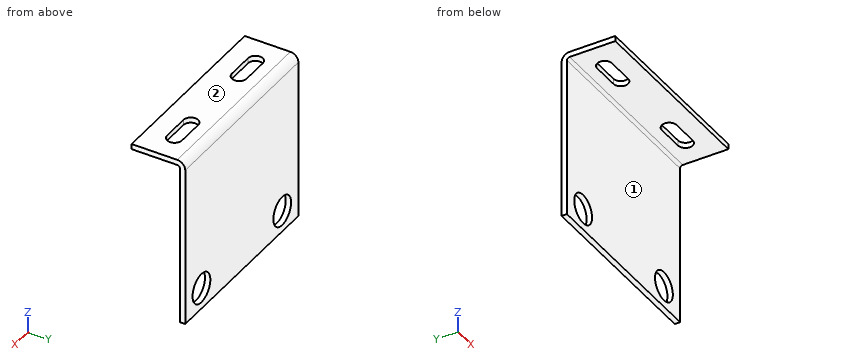
from build123d import *

# Parameters (mm, degrees)
SKETCH_1_W             = 70
SKETCH_1_H             = 60
SM_BASE_FLANGE_1_DEPTH = 2
SM_EDGE_FLANGE_1_DEPTH = 70
CUT_EXTRUDE_1_DEPTH    = 10
SKETCH_13_R            = 5.5
CUT_EXTRUDE_2_DEPTH    = 10


# Sheet-metal steps are written as plain solids
with BuildPart() as part:
    # Sketch 1 → 基体-法兰1 (new body)
    with BuildSketch(Plane(origin=(0, 0, 0), x_dir=(1, 0, 0), z_dir=(0, 1, 0))):
        with Locations((35, 30)):
            Rectangle(SKETCH_1_W, SKETCH_1_H)
    extrude(amount=-SM_BASE_FLANGE_1_DEPTH)

    # 边线-法兰1 section (across the edge) → 边线-法兰1 (add)
    with BuildSketch(Plane(origin=(70, -2, 1), x_dir=(0, 0, -1), z_dir=(-1, 0, 0))):
        with BuildLine():
            Line((-2, 1), (-2, 18))
            Line((-2, 18), (0, 18))
            Line((0, 18), (0, 1))
            ThreePointArc((0, 1), (0.292893219, 0.292893219), (1, 0))
            Line((1, 0), (1, -2))
            ThreePointArc((1, -2), (-1.121320344, -1.121320344), (-2, 1))
        make_face()
    extrude(amount=SM_EDGE_FLANGE_1_DEPTH)

    # 草图12 → 切除-拉伸1 (cut)
    with BuildSketch(Plane(origin=(0, 0, 1), x_dir=(-1, 0, 0), z_dir=(0, 0, -1))):
        with BuildLine():
            Line((-60, -7.25), (-50, -7.25))
            ThreePointArc((-50, -7.25), (-47.25, -10), (-50, -12.75))
            Line((-50, -12.75), (-60, -12.75))
            ThreePointArc((-60, -12.75), (-62.75, -10), (-60, -7.25))
        make_face()
        with BuildLine():
            Line((-10, -7.25), (-20, -7.25))
            ThreePointArc((-20, -7.25), (-22.75, -10), (-20, -12.75))
            Line((-20, -12.75), (-10, -12.75))
            ThreePointArc((-10, -12.75), (-7.25, -10), (-10, -7.25))
        make_face()
    extrude(amount=-CUT_EXTRUDE_1_DEPTH, mode=Mode.SUBTRACT)

    # 草图13 → 切除-拉伸2 (cut)
    with BuildSketch(Plane(origin=(0, 0, 0), x_dir=(1, 0, 0), z_dir=(0, 1, 0))):
        with Locations(Location((10, 52, 0), (0, 0, 270))):
            Circle(SKETCH_13_R)
        with Locations(Location((60, 52, 0), (0, 0, 270))):
            Circle(SKETCH_13_R)
    extrude(amount=-CUT_EXTRUDE_2_DEPTH, mode=Mode.SUBTRACT)


solid = part.part
Could you check a few things on this model? Use its own coordinates, in mm. Face numbers are marked on the shaded views. A direction names the side the tool comes from. Coordinates: 2 decimals unless noted, no trailing zeros. Loops run counter-clockwise (first coordinate to the right, second up) from the corner with the lowest first, then second, coordinate; pieces in that order, holes last.
1. Imagine slicing it at B-B (y = -10). Please give me the cut outline in (x, z).
2. Imagine slicing it at D-D (y = -17.25). Please give me the cut outline in (x, z), and give its area (3 significant figures).
3. Imagine slicing it at C-C (x = 24). Please give me the cut outline in (y, z), and give its area (3 significant figures).
4. Imagine slicing it at A-A (z = -52). Please give me the cut outline in (x, y).
5. For the marked faces 1 and 2, which set-ups out of +Z, -Z, +X, -X, +Y, -Y let a thin tool reach every point of the face, with its end or its side?
6. For P1, Ø8.5, axis at x = 18, y = -7.5, coming from the -Z side; P2, Ø0.6, axis at x = 57, z = 2, coming from the +Y side; P3, Ø6.5, axis at x = 60, z = -52, coming from the +Y side; P4, Ø12.5, axis at x = 10, z = -52, coming from the -Y side, each with a flat end and sliding along its axis, tell me the tip position at first contact or that it passes through.
7. I need wall thicknesses on L1, parallel to X at y = -1.15, z = -52; L2, parallel to Y at x = 61.5, z = -6; L3, parallel to Z at x = 24.5, y = -10.25. Which ranges of each line are inside material? Lowest first, please.
Computed values:
1. outline: (0, 1) - (7.25, 1) - (7.25, 3) - (0, 3) - close; (22.75, 1) - (47.25, 1) - (47.25, 3) - (22.75, 3) - close; (62.75, 1) - (70, 1) - (70, 3) - (62.75, 3) - close
2. outline: (0, 1) - (70, 1) - (70, 3) - (0, 3) - close
2. area: 140 mm2
3. outline: (-20, 1) - (-3, 1) arc R1 cw to (-2, 0) - (-2, -60) - (0, -60) - (0, 0) arc R3 ccw to (-3, 3) - (-20, 3) - close
3. area: 160 mm2
4. outline: (0, -2) - (4.5, -2) - (4.5, 0) - (0, 0) - close; (15.5, -2) - (54.5, -2) - (54.5, 0) - (15.5, 0) - close; (65.5, -2) - (70, -2) - (70, 0) - (65.5, 0) - close
5. face 1: -Z, +X, -X, -Y
5. face 2: +Z, +X, -X, +Y, -Y
6. P1: stops at z = 1
6. P2: stops at y = -0.53
6. P3: passes through
6. P4: stops at y = -2
7. L1: x = 0 to 4.5, 15.5 to 54.5, 65.5 to 70
7. L2: y = -2 to 0
7. L3: z = 1 to 3
